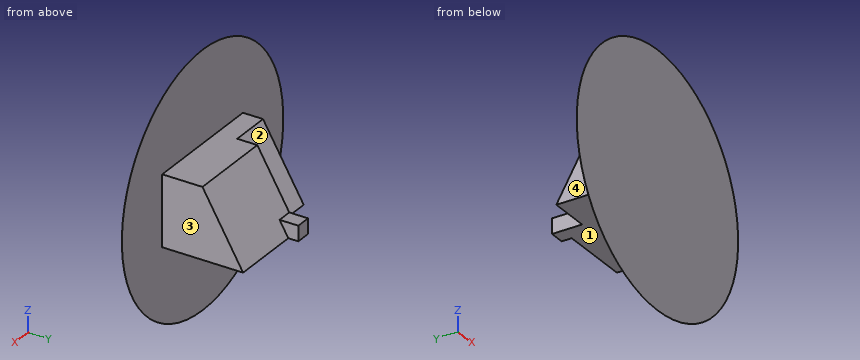
from build123d import *

# Parameters (mm, degrees)
SKETCH1_W           = 125
SKETCH1_H           = 70
EXTRUDE1_DEPTH      = 20
EXTRUDE2_DEPTH      = 40
EXTRUDE3_DEPTH      = 85
SKETCH5_W           = 15
SKETCH5_H           = 15
EXTRUDE5_DEPTH      = 10
EXTRUDE5_DEPTH_BACK = 20
SKETCH6_R           = 125
EXTRUDE6_DEPTH      = 0.01


with BuildPart() as part:
    # Sketch1 → Extrude1 (new body)
    with BuildSketch(Plane(origin=(0, 0, 0), x_dir=(1, 0, 0), z_dir=(0, 1, 0))):
        with Locations((62.5, -35)):
            Rectangle(SKETCH1_W, SKETCH1_H)
    extrude(amount=EXTRUDE1_DEPTH)

    # Sketch2 → Extrude2 (add)
    with BuildSketch(Plane.ZY):
        Polygon((0, 20), (70, 20), (0, 60.414518843), align=None)
    extrude(amount=-EXTRUDE2_DEPTH)

    # Sketch3 → Extrude3 (add)
    with BuildSketch(Plane(origin=(125, 0, 0), x_dir=(0, 0, -1), z_dir=(1, 0, 0))):
        Polygon((-70, 20), (-70, 40), (0, 80.414518843), (0, 20), align=None)
    extrude(amount=-EXTRUDE3_DEPTH)

    # Sketch5 → Extrude5 (add, two sides)
    with BuildSketch(Plane(origin=(0, 80.414518843, 0), x_dir=(-1, 0, 0), z_dir=(0, 1, 0))) as extrude5_sk:
        with Locations((-47.5, 7.5)):
            Rectangle(SKETCH5_W, SKETCH5_H)
    extrude(amount=EXTRUDE5_DEPTH)
    extrude(extrude5_sk.sketch, amount=-EXTRUDE5_DEPTH_BACK)

    # Sketch6 → Extrude6 (add)
    with BuildSketch(Plane(origin=(0, 0, 0), x_dir=(1, 0, 0), z_dir=(0, 1, 0))):
        with Locations(Location((62.5, -35, 0), (0, 0, 270))):  # turned: the seam where the file's is
            Circle(SKETCH6_R)
    extrude(amount=EXTRUDE6_DEPTH)


solid = part.part
Design review of the part built by this model. Coordinates are the model's own, in mm. Face numbers are marked on the shaded views. A direction names the side the tool comes from. Give positions to 0.01 mm unless a question says otherwise; leave off trailing zeros. Loops run counter-clockwise (first coordinate to the right, second up) from the corner with the lowest first, then second, coordinate; pieces in that order, holes last. Notation, with made-up numbers: M 10,58 L 64,58 A23 cw 64,71 Z; hole C 62.5,-8.5 d5. An arc over 180 degrees is marked long. Write item = value, one per line.
Q1. For the marked faces 1, 2, 3 and 4, list the 3-axis set-ups (+Z, -Z, +X, -X, +Y, -Y) from which the entire face can be reached by the end or side of a thin tool; tool diameter is ignored.
Output values:
face_1 = -Z, +X, -X, +Y
face_2 = +Z, -X, +Y
face_3 = +Z, -Z, +X, +Y
face_4 = +Z, -Z, -X, +Y
Q2. We need section C-C (y = 49). Give the boundary of the cut face in (x, z).
Output values:
outline = M 0,0 L 125,0 L 125,54.41 L 40,54.41 L 40,19.77 L 0,19.77 Z
Q3. Insertion check: pin 1 (12 mm diameter, centred on x = 32.5, z = 24, fed in from +Y); pin 2 (1.5 mm diameter, centred on x = 71, y = 58.5, fed in from +Z); pin 3 (12 mm diameter, centred on x = 78.5, y = 24.5, fed in from +Z). Each pin has a flat end and moves straight along its axis. Give the tip position at first contact, or say it passes through.
Output values:
pin_1 = 50.02
pin_2 = 39.26
pin_3 = 70
Q4. To check wall thickness, follow line 1 (Z direction, x = 53, y = 80.5); line 2 (Z direction, x = 9, y = 5); line 3 (Y direction, x = 103, z = 29). State the ranges of each line that lie inside material, in increasing order. Write a range as [from, to].
Output values:
line_1 = [0, 15]
line_2 = [0, 70]
line_3 = [0, 63.67]
